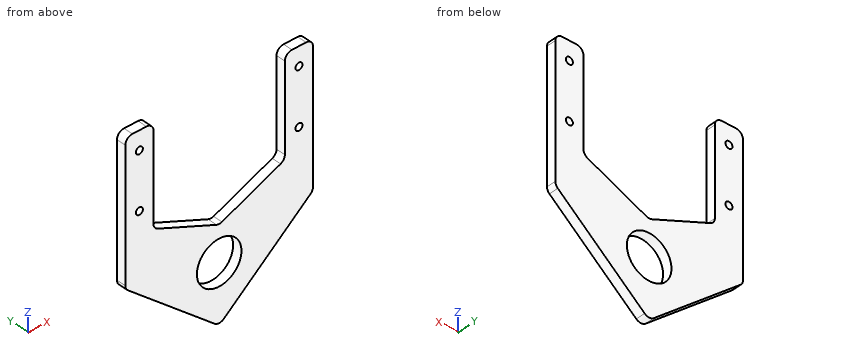
from build123d import *

# Parameters (mm, degrees)
SKETCH_2_R      = 1.5
SKETCH_2_R_2    = 9.5
EXTRUDE_1_DEPTH = 4
FILLET_1_R      = 3


with BuildPart() as part:
    # 草图2 → 凸台-拉伸1 (new body)
    with BuildSketch(Plane(origin=(0, 0, 0), x_dir=(1, 0, 0), z_dir=(0, 1, 0))):
        Polygon((0, 0), (0, 60), (40, 93.908128514), (80, 60), (80, 0), (68, 0), (68, 42), (40, 54), (12, 42), (12, 0), align=None)
        with Locations(Location((6, 32, 0), (0, 0, 270))):
            Circle(SKETCH_2_R, mode=Mode.SUBTRACT)
        with Locations(Location((6, 8, 0), (0, 0, 270))):
            Circle(SKETCH_2_R, mode=Mode.SUBTRACT)
        with Locations(Location((40, 69, 0), (0, 0, 270))):
            Circle(SKETCH_2_R_2, mode=Mode.SUBTRACT)
        with Locations(Location((74, 8, 0), (0, 0, 90))):
            Circle(SKETCH_2_R, mode=Mode.SUBTRACT)
        with Locations(Location((74, 32, 0), (0, 0, 90))):
            Circle(SKETCH_2_R, mode=Mode.SUBTRACT)
    extrude(amount=EXTRUDE_1_DEPTH)

    # 圆角1
    fillet_1_edges = [part.edges().sort_by_distance(p)[0] for p in [
        (0, 2, 0),
        (0, 2, -60),
        (40, 2, -93.908128514),
        (80, 2, -60),
        (80, 2, 0),
        (68, 2, 0),
        (68, 2, -42),
        (40, 2, -54),
        (12, 2, -42),
        (12, 2, 0),
    ]]
    fillet(fillet_1_edges, radius=FILLET_1_R)


solid = part.part
The model under review builds one solid part; all positions refer to its coordinate system, in mm. Coordinates: 2 decimals unless noted, no trailing zeros. Order: outer loops, then holes, each group sorted by start corner. A loop starts at its lowest first (then second) coordinate and runs counter-clockwise, first axis right, second up. Notation, with made-up numbers: (-30.75, 75) -> (-9.75, 75) arc R19 ccw to (-9.75, 104) -> close; hole circle Ø2 at (-21.5, 78.5). An arc over 180 degrees is marked (long way). Answer in a Markdown table with one row per item.
(1) Insertion check: pin 1 (1.8 mm diameter, centred on x = 6, z = -8, fed in from +Y). The pin has a flat end and moves straight along its axis. Give the tip position at first contact, or say it passes through.
Answers:
| item | result |
|---|---|
| pin 1 | through |
(2) Wall thickness on line 1 along X through (y, z) = (0.9, -32); line 2 along X through (y, z) = (3.3, -16); line 3 along Z through (x, y) = (74, 1.1): over which ranges is each line inside the solid? List them lowest first.
Answers:
| item | result |
|---|---|
| line 1 | 0 to 4.5, 7.5 to 12, 68 to 72.5, 75.5 to 80 |
| line 2 | 0 to 12, 68 to 80 |
| line 3 | -65.09 to -33.5, -30.5 to -9.5, -6.5 to 0 |
(3) Consider section A-A (z = -32). Write out the cut boundary in (x, y).
Answers:
| item | result |
|---|---|
| outline | (0, 0) -> (4.5, 0) -> (4.5, 4) -> (0, 4) -> close; (7.5, 0) -> (12, 0) -> (12, 4) -> (7.5, 4) -> close; (68, 0) -> (72.5, 0) -> (72.5, 4) -> (68, 4) -> close; (75.5, 0) -> (80, 0) -> (80, 4) -> (75.5, 4) -> close |
(4) Consider section B-B (y = 1.8). Write out the cut boundary in (x, z).
Answers:
| item | result |
|---|---|
| outline | (0, -58.61) arc R3 ccw to (1.06, -60.9) -> (38.06, -92.26) arc R3 ccw to (41.94, -92.26) -> (78.94, -60.9) arc R3 ccw to (80, -58.61) -> (80, -3) arc R3 ccw to (77, 0) -> (71, 0) arc R3 ccw to (68, -3) -> (68, -40.02) arc R3 cw to (66.18, -42.78) -> (41.18, -53.49) arc R3 cw to (38.82, -53.49) -> (13.82, -42.78) arc R3 cw to (12, -40.02) -> (12, -3) arc R3 ccw to (9, 0) -> (3, 0) arc R3 ccw to (0, -3) -> close; hole circle Ø3 at (6, -32); hole circle Ø3 at (6, -8); hole circle Ø19 at (40, -69); hole circle Ø3 at (74, -32); hole circle Ø3 at (74, -8) |
(5) Consider section D-D (x = 40). Write out the cut boundary in (y, z).
Answers:
| item | result |
|---|---|
| outline | (0, -92.98) -> (4, -92.98) -> (4, -78.5) -> (0, -78.5) -> close; (0, -59.5) -> (4, -59.5) -> (4, -53.74) -> (0, -53.74) -> close |
(6) Consider section C-C (x = 74). Write out the cut boundary in (y, z).
Answers:
| item | result |
|---|---|
| outline | (0, -65.09) -> (4, -65.09) -> (4, -33.5) -> (0, -33.5) -> close; (0, -30.5) -> (4, -30.5) -> (4, -9.5) -> (0, -9.5) -> close; (0, -6.5) -> (4, -6.5) -> (4, 0) -> (0, 0) -> close |
